Work out the finished part from the listing and answer in its coordinate system (mm). Face numbers are marked on the shaded views. A direction names the side the tool comes from. Give positions to 0.01 mm unless a question says otherwise; leave off trailing zeros. Order: outer loops, then holes, each group sorted by start corner. A loop starts at its lowest first (then second) coordinate and runs counter-clockwise, first axis right, second up.
```python
from build123d import *

# Parameters (mm, degrees)
F0_W     = 135.5
F0_H     = 82
F0_R     = 35.5
F1_DEPTH = 1
F2_R     = 36
F4_R     = 23


with BuildPart() as f1:
    # F0 (on Right) → F1 (new body)
    with BuildSketch(Plane.YZ):
        Rectangle(F0_W, F0_H)
        Circle(F0_R, mode=Mode.SUBTRACT)
    extrude(amount=F1_DEPTH)

    # F2 (on face) → F5 section 0
    with BuildSketch(Plane(origin=(0, 0, 0), x_dir=(0, -1, 0), z_dir=(-1, 0, 0))):
        Circle(F2_R)
    # F4 (on offset) → F5 section 1
    with BuildSketch(Plane.YZ.offset(-53)):
        Circle(F4_R)
    loft()


solid = f1.part
```
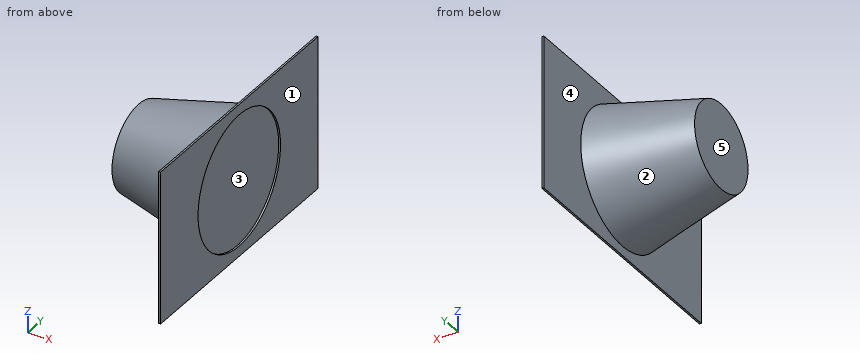
1. The part is cut by section B-B (x = -42.5). Write down the section's boundary in (y, z), then the cut area to 3 significant figures.
Findings below:
outline: circle Ø51.15 at (0, 0)
area: 2,050 mm2
2. Straight lines are drawn through the part: probe 1 along Z at (x, y) = (0.35, 0); probe 2 along X at (y, z) = (-3, 37.5); probe 3 along X at (y, z) = (21, -7.5). For each, find the intervals that lie inside material, in ascending order.
Findings below:
probe 1: z = -41 to -35.5, 35.5 to 41
probe 2: x = 0 to 1
probe 3: x = -53 to 0
3. The mould has two halves that part along Z. Classify the marked faces 1, 2 and 3: pulls with the +Z half, pulls with the -Z half, needs draft (parallel to the pull), parting line crosses it, or undercut.
Findings below:
face 1: needs draft
face 2: parting line crosses it
face 3: undercut
4. Which of the six approach directions +Z, -Z, +X, -X, +Y, -Y give full straight-line access (tool end or side, diameter ignored) to the marked faces 4 and 5?
Findings below:
face 4: -X
face 5: +Z, -Z, -X, +Y, -Y
5. Given P1, Ø5, axis at x = -17.5, y = 7, coming from the -Z side; P2, Ø2, axis at x = -11.5, y = 1.5, coming from the +Z side; P3, Ø6, axis at x = -9, y = -37.5, coming from the -Z side; P4, Ø12, axis at x = -22.5, z = 29.5, coming from the +Y side, each flat-ended and moving along its own axis, determine where each tip first touches the part or whether it passes through.
Findings below:
P1: stops at z = -31.73
P2: stops at z = 33.39
P3: passes through
P4: stops at y = 19.77
6. The part is cut by section A-A (y = 0). Write down the section's boundary in (x, z).
Findings below:
outline: (-53, -23) - (0, -36) - (0, -41) - (1, -41) - (1, -35.5) - (0, -35.5) - (0, 35.5) - (1, 35.5) - (1, 41) - (0, 41) - (0, 36) - (-53, 23) - close
7. The part is cut by section C-C (y = -49.5). Write down the section's boundary in (x, z), then the cut area to 3 significant figures.
Findings below:
outline: (0, -41) - (1, -41) - (1, 41) - (0, 41) - close
area: 82.0 mm2
8. The part is cut by section D-D (x = -2.5). Write down the section's boundary in (y, z), then the cut area to 3 significant figures.
Findings below:
outline: circle Ø70.77 at (0, 0)
area: 3,930 mm2
